For this review, take the finished solid that the model builds, in its own axes (mm). A direction names the side the tool comes from. Round coordinates to 2 decimals unless told otherwise and drop trailing zeros. Write each loop counter-clockwise with the first axis right and the second up, starting at its lowest first coordinate (ties: lowest second). Pieces come first, ordered by that corner, then holes.
from build123d import *

# Parameters (mm, degrees)
F0_W      = 100
F0_H      = 100
F1_DEPTH  = 50
F2_R      = 5
F3_R      = 5
F4_R      = 20
F5_DEPTH  = 5
F6_R      = 9
F7_DEPTH  = 5
F8_R      = 12
F9_DEPTH  = 5
F10_R     = 12
F11_DEPTH = 5
F12_R     = 15
F13_DEPTH = 2
F14_R     = 12
F15_DEPTH = 5


with BuildPart() as f1:
    # F0 (on Front) → F1 (new body, symmetric)
    with BuildSketch(Plane.XZ):
        Rectangle(F0_W, F0_H)
    extrude(amount=F1_DEPTH, both=True)

    # F2
    f2_edges = [f1.edges().sort_by_distance(p)[0] for p in [
        (0, -50, 50),
        (0, 50, -50),
        (0, -50, -50),
        (0, 50, 50),
    ]]
    fillet(f2_edges, radius=F2_R)

    # F3
    f3_edges = [f1.edges().sort_by_distance(p)[0] for p in [
        (50, 0, 50),
        (-50, 0, 50),
    ]]
    fillet(f3_edges, radius=F3_R)

    # F4 (on face) → F5 (cut)
    with BuildSketch(Plane.XY.offset(50)):
        Circle(F4_R)
    extrude(amount=-F5_DEPTH, mode=Mode.SUBTRACT)

    # F6 (on face) → F7 (cut)
    with BuildSketch(Plane(origin=(0, 0, -50), x_dir=(1, 0, 0), z_dir=(0, 0, -1))):
        with Locations((-24, -24)):
            Circle(F6_R)
        with Locations((-24, 24)):
            Circle(F6_R)
        with Locations((-24, 0)):
            Circle(F6_R)
        with Locations((24, 24)):
            Circle(F6_R)
        with Locations((24, 0)):
            Circle(F6_R)
        with Locations((24, -24)):
            Circle(F6_R)
    extrude(amount=-F7_DEPTH, mode=Mode.SUBTRACT)

    # F8 (on face) → F9 (cut)
    with BuildSketch(Plane.XZ.offset(50)):
        with Locations((-24, 24)):
            Circle(F8_R)
        Circle(F8_R)
        with Locations((24, -24)):
            Circle(F8_R)
    extrude(amount=-F9_DEPTH, mode=Mode.SUBTRACT)

    # F10 (on face) → F11 (cut)
    with BuildSketch(Plane(origin=(0, 50, 0), x_dir=(-1, 0, 0), z_dir=(0, 1, 0))):
        with Locations((24, 24)):
            Circle(F10_R)
        with Locations((-24, 24)):
            Circle(F10_R)
        with Locations((24, -24)):
            Circle(F10_R)
        with Locations((-24, -24)):
            Circle(F10_R)
    extrude(amount=-F11_DEPTH, mode=Mode.SUBTRACT)

    # F12 (on face) → F13 (cut)
    with BuildSketch(Plane.YZ.offset(50)):
        with Locations((-24, 24)):
            Circle(F12_R)
        with Locations((24, -24)):
            Circle(F12_R)
    extrude(amount=-F13_DEPTH, mode=Mode.SUBTRACT)

    # F14 (on face) → F15 (cut)
    with BuildSketch(Plane(origin=(-50, 0, 0), x_dir=(0, -1, 0), z_dir=(-1, 0, 0))):
        with Locations((-26, 26)):
            Circle(F14_R)
        with Locations((26, 26)):
            Circle(F14_R)
        Circle(F14_R)
        with Locations((-26, -26)):
            Circle(F14_R)
        with Locations((26, -26)):
            Circle(F14_R)
    extrude(amount=-F15_DEPTH, mode=Mode.SUBTRACT)


solid = f1.part
(1) We need section B-B, the plane y = 0. Give the boundary of the cut face in (x, z), and give its area (3 significant figures).
Geometry check:
outline: (-50, -45) arc R5 ccw to (-45, -50) - (-33, -50) - (-33, -45) - (-15, -45) - (-15, -50) - (15, -50) - (15, -45) - (33, -45) - (33, -50) - (45, -50) arc R5 ccw to (50, -45) - (50, 45) arc R5 ccw to (45, 50) - (20, 50) - (20, 45) - (-20, 45) - (-20, 50) - (-45, 50) arc R5 ccw to (-50, 45) - (-50, 12) - (-45, 12) - (-45, -12) - (-50, -12) - close
area: 9,480 mm2
(2) We need section C-C, the plane x = 0. Give the boundary of the cut face in (y, z).
Geometry check:
outline: (-50, -45) arc R5 ccw to (-45, -50) - (45, -50) arc R5 ccw to (50, -45) - (50, 45) arc R5 ccw to (45, 50) - (20, 50) - (20, 45) - (-20, 45) - (-20, 50) - (-45, 50) arc R5 ccw to (-50, 45) - (-50, 12) - (-45, 12) - (-45, -12) - (-50, -12) - close
(3) We need section A-A, the plane z = 0. Give the boundary of the cut face in (x, y).
Geometry check:
outline: (-50, -45) arc R5 ccw to (-45, -50) - (-12, -50) - (-12, -45) - (12, -45) - (12, -50) - (45, -50) arc R5 ccw to (50, -45) - (50, 45) arc R5 ccw to (45, 50) - (-45, 50) arc R5 ccw to (-50, 45) - (-50, 12) - (-45, 12) - (-45, -12) - (-50, -12) - close
(4) For line 1 along Y through (x, z) = (24, -47.6); line 2 along Z through (x, y) = (-24, 48); line 3 along Y through (x, z) = (24, -48.65), list the stretches that pass through material, from the lowest coordinate up.
Geometry check:
line 1: y = -49.27 to -33, -15 to -9, 9 to 15, 33 to 49.27
line 2: z = -49 to -36, -12 to 12, 36 to 49
line 3: y = -48.42 to -33, -15 to -9, 9 to 15, 33 to 48.42
(5) Mouldability with a two-part tool opening along X and no side actions: class faces 1 (the face through (-1, -21, 50)), 2 (the face through (24, -45, -24)), 3 (the face through (-49, -1, -48)), 4 (the face through (-15.416, 21.297, -47.535)) as pulls with the +X half, pulls with the -X half, needs draft (parallel to the pull), parting line crosses it, or undercut.
Geometry check:
face 1: needs draft
face 2: undercut
face 3: pulls with the -X half
face 4: undercut
(6) For pin 1 Ø5.5 at (x, y) = (-28.5, -1.5) entering from -Z; pin 2 Ø19 at (x, z) = (24, -24) entering from +Y; pin 3 Ø18 at (y, z) = (-24, 24) entering from +X, all flat-tipped, find the tip position at first contact; note any pin that passes through.
Geometry check:
pin 1: stops at z = -45
pin 2: stops at y = 45
pin 3: stops at x = 48
(7) For faces 5 (the face through (24, -24, -45)), 6 (the face through (-49, -48, 1)), 7 (the face through (49.014, -27.252, 9.357)), 8 (the face through (-45, -26, 26)), 9 (the face through (-1, 50, 1)), list the 3-axis set-ups (+Z, -Z, +X, -X, +Y, -Y) from which the entire face can be reached by the end or side of a thin tool; tool diameter is ignored.
Geometry check:
face 5: -Z
face 6: +Z, -Z, -X, -Y
face 7: +X
face 8: -X
face 9: +Z, -Z, +X, -X, +Y
